```python
from build123d import *

# Parameters (mm, degrees)
SKETCH1_R           = 3.95
BOSS_EXTRUDE1_DEPTH = 12
SKETCH2_W           = 5.25
SKETCH2_H           = 5.25
BOSS_EXTRUDE2_DEPTH = 10
CUT_EXTRUDE1_DEPTH  = 11
FILLET1_R           = 0.75
FILLET2_R           = 0.4


with BuildPart() as part:
    # Sketch1 → Boss-Extrude1 (new body)
    with BuildSketch(Plane(origin=(0, 0, 0), x_dir=(1, 0, 0), z_dir=(0, 1, 0))):
        with Locations(Location((0, 0, 0), (0, 0, 270))):
            Circle(SKETCH1_R)
    extrude(amount=BOSS_EXTRUDE1_DEPTH)

    # Sketch2 → Boss-Extrude2 (add)
    with BuildSketch(Plane(origin=(0, 12, 0), x_dir=(1, 0, 0), z_dir=(0, 1, 0))):
        Rectangle(SKETCH2_W, SKETCH2_H)
    extrude(amount=BOSS_EXTRUDE2_DEPTH)

    # Sketch3 → Cut-Extrude1 (cut)
    with BuildSketch(Plane.XZ):
        with BuildLine():
            Line((1.025, -1.540089283), (-1.025, -1.540089283))
            ThreePointArc((-1.025, -1.540089283), (0, 1.85), (1.025, -1.540089283))
        make_face()
    extrude(amount=-CUT_EXTRUDE1_DEPTH, mode=Mode.SUBTRACT)

    # Fillet1
    fillet1_edges = [part.edges().sort_by_distance(p)[0] for p in [
        (-2.625, 17, -2.625),
        (-2.625, 17, 2.625),
        (2.625, 17, 2.625),
        (2.625, 17, -2.625),
    ]]
    fillet(fillet1_edges, radius=FILLET1_R)

    # Fillet2
    fillet2_edges = [part.edges().sort_by_distance(p)[0] for p in [
        (0, 0, 1.85),
        (0, 0, -1.540089283),
        (0, 0, -3.95),
        (2.625, 22, 0),
        (0, 22, 2.625),
        (-2.625, 22, 0),
        (0, 22, -2.625),
        (-2.405330086, 22, 2.405330086),
        (-2.405330086, 22, -2.405330086),
        (2.405330086, 22, -2.405330086),
        (2.405330086, 22, 2.405330086),
        (0, 12, -3.95),
    ]]
    fillet(fillet2_edges, radius=FILLET2_R)


solid = part.part
```
The model under review builds one solid part; all positions refer to its coordinate system, in mm. A direction names the side the tool comes from. Round coordinates to 2 decimals unless told otherwise and drop trailing zeros. Order: outer loops, then holes, each group sorted by start corner. A loop starts at its lowest first (then second) coordinate and runs counter-clockwise, first axis right, second up. Notation, with made-up numbers: (68.5, 67) - (96.5, 67) arc R32 ccw to (96.5, 102) - close; hole circle Ø3 at (-14.5, 9). An arc over 180 degrees is marked (long way). Answer in a Markdown table with one row per item.
(1) Clearance check with flat-ended pins moving along their axes: P1, Ø1.1, axis at x = 0.5, y = 15, coming from the +Z side (3 decimals); P2, Ø4, axis at x = 0.5, y = 17, coming from the -Z side (3 decimals); P3, Ø2, axis at x = -0.5, z = 0, coming from the -Y side. State where each tip first meets the part, or that it passes through.
Result set:
| item | result |
|---|---|
| P1 | stops at z = 2.625 |
| P2 | stops at z = -2.625 |
| P3 | stops at y = 11 |
(2) Take a section at A-A on y = 15.25. Write out the cut boundary in (x, z) (3 decimals).
Result set:
| item | result |
|---|---|
| outline | (-2.625, -1.875) arc R0.75 ccw to (-1.875, -2.625) - (1.875, -2.625) arc R0.75 ccw to (2.625, -1.875) - (2.625, 1.875) arc R0.75 ccw to (1.875, 2.625) - (-1.875, 2.625) arc R0.75 ccw to (-2.625, 1.875) - close |
(3) Machinability: for faces 1 (the face through (0, 6, -1.54)), 2 (the face through (3, 12, 0)), 3 (the face through (-2.625, 17, 0)), which of the approach directions +Z, -Z, +X, -X, +Y, -Y give a long, thin tool a straight path to every point of the face, cutting with its end or side? Answer none if there is none.
Result set:
| item | result |
|---|---|
| face 1 | -Y |
| face 2 | +Y |
| face 3 | +Z, -Z, -X, +Y |
(4) Take a section at B-B on x = 0. Write out the cut boundary in (y, z) (3 decimals).
Result set:
| item | result |
|---|---|
| outline | (0, -3.55) arc R0.4 ccw to (0.4, -3.95) - (11.6, -3.95) arc R0.4 ccw to (12, -3.55) - (12, -2.625) - (21.6, -2.625) arc R0.4 ccw to (22, -2.225) - (22, 2.225) arc R0.4 ccw to (21.6, 2.625) - (12, 2.625) - (12, 3.55) arc R0.4 ccw to (11.6, 3.95) - (0.4, 3.95) arc R0.4 ccw to (0, 3.55) - (0, 2.25) arc R0.4 ccw to (0.4, 1.85) - (11, 1.85) - (11, -1.54) - (0.4, -1.54) arc R0.4 ccw to (0, -1.94) - close |
(5) Mouldability with a two-part tool opening along Z and no side actions: class faces 4 (the face through (0, 11, 0)), 5 (the face through (0, 17, -2.625)), 6 (the face through (0, 17, 2.625)), 7 (the face through (0, 22, 0)) as released by +Z, released by -Z, zero draft, split by the parting line, or undercut.
Result set:
| item | result |
|---|---|
| face 4 | undercut |
| face 5 | released by -Z |
| face 6 | released by +Z |
| face 7 | zero draft |
(6) For line 1 (X direction, y = 4.75, z = 0); line 2 (Z direction, x = 0.25, y = 17.5) (3 decimals); line 3 (Y direction, x = 0.75, z = 3.25), list the stretches that pass through material, from the lowest coordinate up. Write a range as from..to.
Result set:
| item | result |
|---|---|
| line 1 | x = -3.95..-1.85, 1.85..3.95 |
| line 2 | z = -2.625..2.625 |
| line 3 | y = 0..12 |
